```python
from build123d import *

# Parameters (mm, degrees)
BOSS_EXTRUDE1_DEPTH = 25.4
SKETCH2_W           = 44.547462604
SKETCH2_H           = 25.4
BOSS_EXTRUDE2_DEPTH = 12.7
SKETCH3_W           = 22.225
SKETCH3_H           = 22.225
BOSS_EXTRUDE3_DEPTH = 19.05
SKETCH4_W           = 22.225
SKETCH4_H           = 22.225
BOSS_EXTRUDE4_DEPTH = 19.05
SKETCH5_W           = 22.225
SKETCH5_H           = 22.225
BOSS_EXTRUDE5_DEPTH = 19.05
BOSS_EXTRUDE6_DEPTH = 19.05
CUT_EXTRUDE1_DEPTH  = 580.024222363


with BuildPart() as part:
    # Sketch1 → Boss-Extrude1 (new body)
    with BuildSketch(Plane(origin=(0, 0, 0), x_dir=(1, 0, 0), z_dir=(0, 1, 0))):
        with BuildLine():
            Line((-476.965634664, 197.565634664), (-436.048451995, 238.482817332))
            Line((-436.048451995, 238.482817332), (-454.008964237, 256.443329574))
            ThreePointArc((-454.008964237, 256.443329574), (-489.798145481, 202.881034683), (-502.365634664, 139.7))
            Line((-502.365634664, 139.7), (-476.965634664, 139.7))
            Line((-476.965634664, 139.7), (-476.965634664, 197.565634664))
        make_face()
        with BuildLine():
            ThreePointArc((-476.965634664, 139.7), (-466.331605355, 193.160875501), (-436.048451995, 238.482817332))
            Line((-436.048451995, 238.482817332), (-476.965634664, 197.565634664))
            Line((-476.965634664, 197.565634664), (-476.965634664, 139.7))
        make_face()
    extrude(amount=BOSS_EXTRUDE1_DEPTH)

    # Sketch2 → Boss-Extrude2 (add, symmetric)
    with BuildSketch(Plane(origin=(0, 0, 0), x_dir=(0.9238795325112892, 0, 0.3826834323650839), z_dir=(-0.3826834323650839, 0, 0.9238795325112892))):
        Polygon((-504.753692386, 0), (-530.153692386, 0), (-530.153692386, -12.7), (-512.779069106, -60.436385136), (-488.910876538, -51.749073495), (-498.50115499, -25.4), (-498.50115499, 0), align=None)
        with Locations((-476.227423688, -12.7)):
            Rectangle(SKETCH2_W, SKETCH2_H)
    extrude(amount=BOSS_EXTRUDE2_DEPTH, both=True)

    # Sketch3 → Boss-Extrude3 (add)
    with BuildSketch(Plane.XY.offset(-139.7)):
        with Locations((-489.665634664, 12.7)):
            Rectangle(SKETCH3_W, SKETCH3_H)
    extrude(amount=BOSS_EXTRUDE3_DEPTH)

    # Sketch4 → Boss-Extrude4 (add)
    with BuildSketch(Plane(origin=(-98.782817332, 0, 98.782817332), x_dir=(-0.7071067811865343, 0, -0.7071067811865608), z_dir=(0.7071067811865608, 0, -0.7071067811865343))):
        with Locations((489.665634664, 12.7)):
            Rectangle(SKETCH4_W, SKETCH4_H)
    extrude(amount=BOSS_EXTRUDE4_DEPTH)

    # Sketch5 → Boss-Extrude5 (add)
    with BuildSketch(Plane(origin=(-419.398525104, 0, -173.720557137), x_dir=(0.3826834323650839, 0, -0.9238795325112892), z_dir=(0.9238795325112892, 0, 0.3826834323650839))):
        with Locations((0, -12.7)):
            Rectangle(SKETCH5_W, SKETCH5_H)
    extrude(amount=BOSS_EXTRUDE5_DEPTH)

    # Sketch6 → Boss-Extrude6 (add)
    with BuildSketch(Plane(origin=(-37.4724398, 111.437344998, -15.52159278), x_dir=(0.9487640489542349, 0.3129641753372822, -0.043591333627466894), z_dir=(0.31598541012516107, -0.9396926207859091, 0.13088544238586405))):
        Polygon((-462.863246728, -191.884470829), (-453.898805786, -212.221368911), (-433.561907704, -203.25692797), (-442.526348645, -182.920029887), align=None)
    extrude(amount=BOSS_EXTRUDE6_DEPTH)

    # Sketch7 → Cut-Extrude1 (cut, through all)
    with BuildSketch(Plane(origin=(0, 25.4, 0), x_dir=(1, 0, 0), z_dir=(0, 1, 0))):
        with BuildLine():
            ThreePointArc((-494.206275899, 190.960561143), (-492.116958141, 196.963230937), (-489.798145481, 202.881034683))
            Line((-489.798145481, 202.881034683), (-494.658225072, 191.147764621))
            Line((-494.658225072, 191.147764621), (-494.206275899, 190.960561143))
        make_face()
        with BuildLine():
            Line((-484.486116716, 214.427101269), (-484.93806589, 214.614304746))
            Line((-484.93806589, 214.614304746), (-489.798145481, 202.881034683))
            ThreePointArc((-489.798145481, 202.881034683), (-487.253274478, 208.705201999), (-484.486116716, 214.427101269))
        make_face()
    extrude(amount=-CUT_EXTRUDE1_DEPTH, mode=Mode.SUBTRACT)


solid = part.part
```
Input: part model. Units: mm. Frame: model coordinates. A direction names the side the tool comes from. Give positions to 0.01 mm unless a question says otherwise; leave off trailing zeros. Write each loop counter-clockwise with the first axis right and the second up, starting at its lowest first coordinate (ties: lowest second). Pieces come first, ordered by that corner, then holes. Notation, with made-up numbers: (76.5, -9) - (108.5, -9) arc R5 cw to (108.5, -3) - close; hole circle Ø2 at (72.5, 22). An arc over 180 degrees is marked (long way). Write item = value, one per line. Start each with the question number.
1. Section query B-B, the plane z = -160. Output: boundary loops of the cut face in (x, y).
2. Ray query, L1, parallel to Y at x = -451, z = -249; L2, parallel to X at y = -30, z = -201; L3, parallel to X at y = -18, z = -163.5. Return the intervals inside material, ascending.
3. Section query C-C, the plane x = -427.5. Output: boundary loops of the cut face in (y, z), then the cut area to 3 significant figures.
4. Mould query, pull axis Y, two halves, no side actions, for faces 6 (the flat face through (-446.25, 12.54, -261.96)), 7 (the flat face through (-456.13, -38.76, -188.74)), 8 (the flat face through (-438, 23.812, -254)), 9 (the flat face through (-487, 0, -166)). Classes: released by +Y, released by -Y, zero draft, split by the parting line, or undercut.
5. Section query D-D, the plane x = -487.5. Output: boundary loops of the cut face in (y, z), then the cut area to 3 significant figures.
6. Section query A-A, the plane y = 8. Output: boundary loops of the cut face in (x, z).
7. First-contact query: pin 1 Ø5.5 at (x, z) = (-487.5, -130.5) entering from -Y; pin 2 Ø9.5 at (x, z) = (-482.5, -173.5) entering from -Y; pin 3 Ø13 at (x, z) = (-413.5, -176) entering from -Y. Flat tips, straight axial feed; report the tip coordinate or a pass-through.
8. Access query for faces 1 (the flat face through (-478.553, 13, -130)), 2 (the flat face through (-411, -23.812, -170)), 3 (the flat face through (-472.595, -59.974, -195.691)), 4 (the cylindrical face through (-466.624, 12.522, -192.45)), 5 (the flat face through (-450.046, -61.117, -186.583)). Directions: +Z, -Z, +X, -X, +Y, -Y. A direction counts if a zero-diameter tool reaches every point of the face in a straight line with its end or side. Return the directions, or none.
Check sheet entries:
q1.outline = (-501.11, 0) - (-475.48, 0) - (-475.48, 25.4) - (-501.11, 25.4) - close; (-415.31, -23.81) - (-404.46, -23.81) - (-404.46, -1.59) - (-415.31, -1.59) - close
q2.L1 = 0 to 25.4
q2.L2 = -483.76 to -454.5
q2.L3 = -427.91 to -403.01
q3.outline = (-25.4, -190.82) - (0, -190.82) - (0, -163.33) - (-25.4, -163.33) - close; (1.59, -256.88) - (23.81, -256.88) - (23.81, -249.28) - (1.59, -249.28) - close
q3.area = 867 mm2
q4.face_6 = zero draft
q4.face_7 = undercut
q4.face_8 = released by +Y
q4.face_9 = released by -Y
q5.outline = (-33.99, -188.18) - (-12.98, -208.17) - (25.4, -208.17) - (25.4, -139.7) - (23.81, -139.7) - (23.81, -120.65) - (1.59, -120.65) - (1.59, -139.7) - (0, -139.7) - (0, -188.18) - close
q5.area = 2,630 mm2
q6.outline = (-502.37, -139.7) arc R165.1 ccw to (-454.01, -256.44) - (-452.89, -255.32) - (-439.42, -268.79) - (-423.7, -253.08) - (-437.17, -239.61) - (-436.05, -238.48) arc R139.7 cw to (-476.97, -139.7) - (-478.55, -139.7) - (-478.55, -120.65) - (-500.78, -120.65) - (-500.78, -139.7) - close
q7.pin_1 = 1.59
q7.pin_2 = 0
q7.pin_3 = -25.4
q8.face_1 = +Z, +X, +Y, -Y
q8.face_2 = +Z, +X, -Y
q8.face_3 = none
q8.face_4 = +Z, +X, +Y
q8.face_5 = +Z, +X
